Source: three-view drawing plus pictorial views. Frame: mm from the lowest corner of the part. A direction names the side the tool comes from. Give positions to 0.01 mm unless a question says otherwise; leave off trailing zeros. Write each loop counter-clockwise with the first axis right and the second up, starting at its lowest first coordinate (ties: lowest second). Pieces come first, ordered by that corner, then holes.
Q1. Line query: L1, parallel to Z at x = 4.25, y = 6.75; L2, parallel to Y at x = 4.25, z = 41.5; L3, parallel to Z at x = 4.25, y = 31. Output: solid intervals per line, ascending.
Q2. Cut plane B-B on y = 28. Return the cut outline in (x, z).
Q3. Reachability of the marked faces 1 and 2 from +Z, -Z, +X, -X, +Y, -Y: full face, straight path, thin tool, end or side. Return the list, or none.
Q4. Pin query (flat end, axial travel): pin 1 (4 mm diameter, centred on x = 2.5, y = 23, fed in from -Z); pin 2 (5 mm diameter, centred on x = 1.5, z = 5.5, fed in from +Y); pin 3 (4 mm diameter, centred on x = 4.25, z = 18, fed in from -Y) (3 decimals). Return the tip coordinate at first contact, or that it passes through.
Q5. Cut plane D-D on z = 40.5. Return the cut outline in (x, y).
Q6. Cut plane A-A on x = 4.25. Return the cut outline in (y, z), plus the area to 3 significant figures.
Q7. Cut plane C-C on z = 18.5. Return the cut outline in (x, y), plus the area to 3 significant figures.
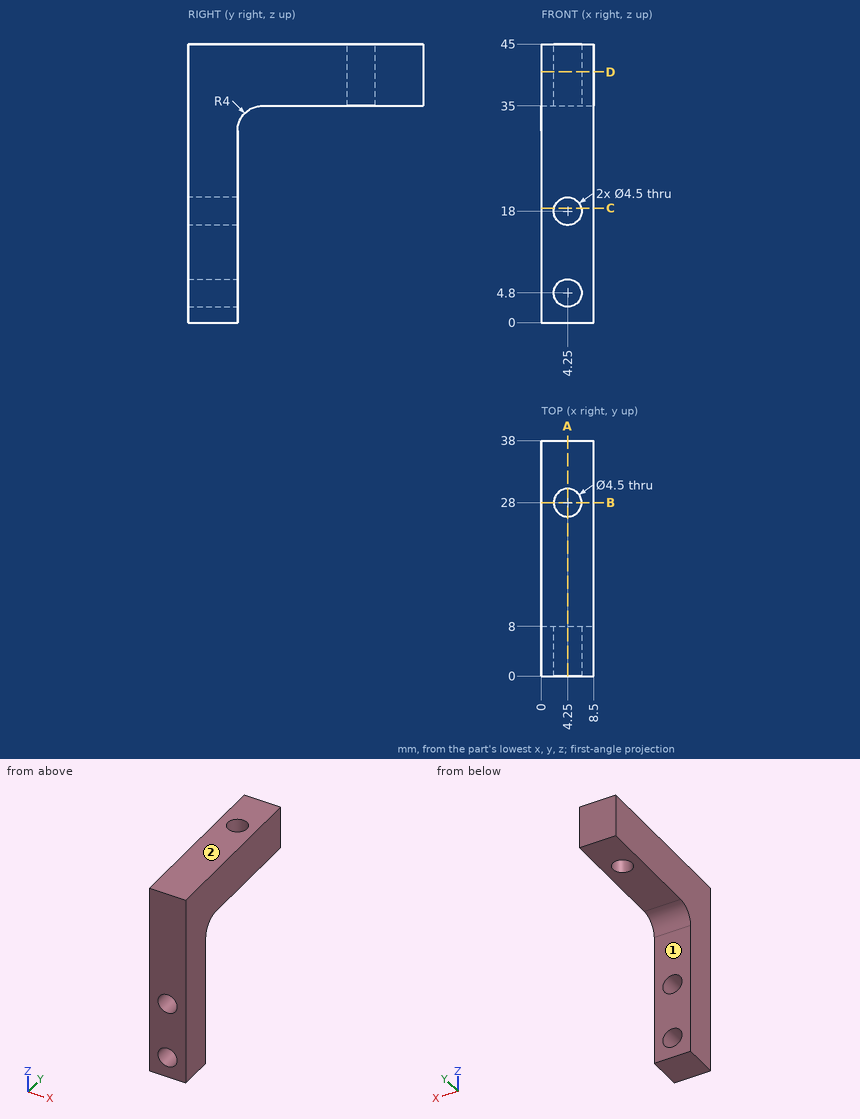
Data:
1. L1: z = 0 to 2.55, 7.05 to 15.75, 20.25 to 45
1. L2: y = 0 to 25.75, 30.25 to 38
1. L3: z = 35 to 45
2. outline: (0, 35) - (2, 35) - (2, 45) - (0, 45) - close; (6.5, 35) - (8.5, 35) - (8.5, 45) - (6.5, 45) - close
3. face 1: -Z, +X, -X, +Y
3. face 2: +Z, +X, -X, +Y, -Y
4. pin 1: stops at z = 35
4. pin 2: stops at y = 8
4. pin 3: passes through
5. outline: (0, 0) - (8.5, 0) - (8.5, 38) - (0, 38) - close; hole circle Ø4.5 at (4.25, 28)
6. outline: (0, 0) - (8, 0) - (8, 2.55) - (0, 2.55) - close; (0, 7.05) - (8, 7.05) - (8, 15.75) - (0, 15.75) - close; (0, 20.25) - (8, 20.25) - (8, 31) arc R4 cw to (12, 35) - (25.75, 35) - (25.75, 45) - (0, 45) - close; (30.25, 35) - (38, 35) - (38, 45) - (30.25, 45) - close
6. area: 546 mm2
7. outline: (0, 0) - (2.06, 0) - (2.06, 8) - (0, 8) - close; (6.44, 0) - (8.5, 0) - (8.5, 8) - (6.44, 8) - close
7. area: 32.9 mm2
